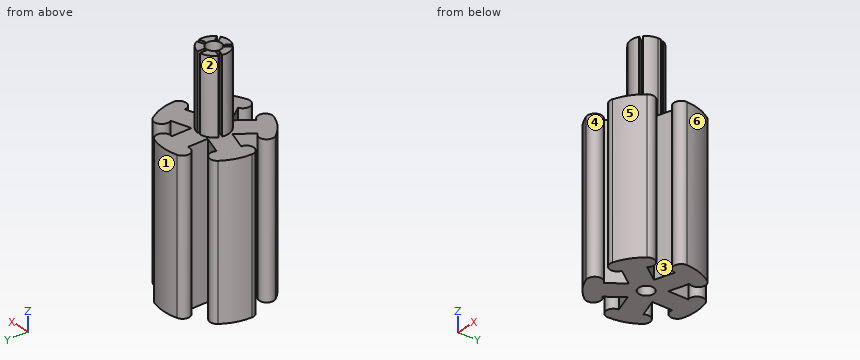
```python
from build123d import *

# Parameters (mm, degrees)
BOSS_EXTRUDE3_DEPTH = 30
CIRPATTERN1_COUNT   = 5
BOSS_EXTRUDE4_DEPTH = 15
SKETCH6_R           = 1.5
CUT_EXTRUDE1_DEPTH  = 80


with BuildPart() as part:
    # Sketch2 → Boss-Extrude3 (new body)
    with BuildSketch(Plane.XY):
        with BuildLine():
            Line((-2.054029869, 6.78303703), (-2.054029869, 0))
            Line((-2.054029869, 0), (2.054029869, 0))
            Line((2.054029869, 0), (2.054029869, 6.78303703))
            ThreePointArc((2.054029869, 6.78303703), (3.825708627, 7.801903653), (2.835284544, 9.589638239))
            ThreePointArc((2.835284544, 9.589638239), (0, 10), (-2.835284544, 9.589638239))
            ThreePointArc((-2.835284544, 9.589638239), (-3.825708627, 7.801903653), (-2.054029869, 6.78303703))
        make_face()
    extrude(amount=-BOSS_EXTRUDE3_DEPTH)

    # CirPattern1: part ×5 about axis
    cirpattern1_axis = Axis((0, 0, 0), (0, 0, 1))


with BuildPart() as part_1:
    add(part.part)
    for i in range(1, CIRPATTERN1_COUNT):
        add(part.part.rotate(cirpattern1_axis, i * 360 / CIRPATTERN1_COUNT))

    # Sketch7 → Boss-Extrude4 (add)
    with BuildSketch(Plane.XY):
        with BuildLine():
            Line((0.3, 2.984962311), (0.3, 1.687380928))
            Line((0.3, 1.687380928), (-0.3, 1.687380928))
            Line((-0.3, 1.687380928), (-0.3, 2.984962311))
            ThreePointArc((-0.3, 2.984962311), (-1.763355757, 2.427050983), (-2.746162759, 1.207721037))
            Line((-2.746162759, 1.207721037), (-1.512089528, 0.806746337))
            Line((-1.512089528, 0.806746337), (-1.697499725, 0.236112428))
            Line((-1.697499725, 0.236112428), (-2.931572955, 0.637087127))
            ThreePointArc((-2.931572955, 0.637087127), (-2.853169549, -0.927050983), (-1.997221924, -2.238549662))
            Line((-1.997221924, -2.238549662), (-1.234522723, -1.188784271))
            Line((-1.234522723, -1.188784271), (-0.749112526, -1.541455422))
            Line((-0.749112526, -1.541455422), (-1.511811727, -2.591220813))
            ThreePointArc((-1.511811727, -2.591220813), (0, -3), (1.511811727, -2.591220813))
            Line((1.511811727, -2.591220813), (0.749112526, -1.541455422))
            Line((0.749112526, -1.541455422), (1.234522723, -1.188784271))
            Line((1.234522723, -1.188784271), (1.997221924, -2.238549662))
            ThreePointArc((1.997221924, -2.238549662), (2.737851874, -1.226444909), (3, 0))
            ThreePointArc((3, 0), (2.982844185, 0.320375665), (2.931572955, 0.637087127))
            Line((2.931572955, 0.637087127), (1.697499725, 0.236112428))
            Line((1.697499725, 0.236112428), (1.512089528, 0.806746337))
            Line((1.512089528, 0.806746337), (2.746162759, 1.207721037))
            ThreePointArc((2.746162759, 1.207721037), (1.763355757, 2.427050983), (0.3, 2.984962311))
        make_face()
    extrude(amount=BOSS_EXTRUDE4_DEPTH)

    # Sketch6 → Cut-Extrude1 (cut)
    with BuildSketch(Plane(origin=(0, 0, -30), x_dir=(-1, 0, 0), z_dir=(0, 0, -1))):
        Circle(SKETCH6_R)
    extrude(amount=-CUT_EXTRUDE1_DEPTH, mode=Mode.SUBTRACT)


solid = part_1.part
```
Input: part model. Units: mm. Frame: model coordinates. Face numbers are marked on the shaded views. A direction names the side the tool comes from. Coordinates: 2 decimals unless noted, no trailing zeros. Order: outer loops, then holes, each group sorted by start corner. A loop starts at its lowest first (then second) coordinate and runs counter-clockwise, first axis right, second up. Notation, with made-up numbers: (52.5, 88) - (72.5, 88) arc R11 cw to (72.5, 101) - close; hole circle Ø6 at (-29.5, -12.75). An arc over 180 degrees is marked (long way). Put each result on its own line as item: value.
1. Line query: line 1 along Z through (x, y) = (5, 0.5); line 2 along X through (y, z) = (-4, -23.5); line 3 along Y through (x, z) = (3.25, -10). Output: solid intervals per line, ascending.
Report:
line 1: z = -30 to 0
line 2: x = -7.6 to -5.96, -5.45 to -0.37, 0.37 to 5.45, 5.96 to 7.6
line 3: y = -9.45 to 3.22, 6.99 to 9.39
2. Cut plane C-C on y = 7.25. Return the cut outline in (x, z), then the cut area to 3 significant figures.
Report:
outline: (-3.53, -30) - (3.53, -30) - (3.53, 0) - (-3.53, 0) - close
area: 212 mm2
3. Reachability of the marked faces 1, 2 and 3 from +Z, -Z, +X, -X, +Y, -Y: full face, straight path, thin tool, end or side. Return the list, or none.
Report:
face 1: +Z, -Z, +Y
face 2: +Z, -X, +Y
face 3: +Z, -Z
4. Cut plane D-D on x = 8.75. Return the cut outline in (y, z), then the cut area to 3 significant figures.
Report:
outline: (-1.21, -30) - (4.84, -30) - (4.84, 0) - (-1.21, 0) - close
area: 182 mm2
5. Contact query for flat-ended pins moving along their axis: pin 1 Ø10 at (x, z) = (6.5, -13.5) entering from +Y; pin 2 Ø3 at (y, z) = (5.5, -8) entering from -X; pin 3 Ø1 at (y, z) = (2.5, 9) entering from -X. Output: stop coordinate, or through.
Report:
pin 1: stops at y = 9.89
pin 2: stops at x = -9.17
pin 3: stops at x = -2.24
6. Cut plane A-A on z = 5. Return the cut outline in (x, y), then the cut area to 3 significant figures.
Report:
outline: (-2.93, 0.64) arc R3 ccw to (-2, -2.24) - (-1.23, -1.19) - (-0.75, -1.54) - (-1.51, -2.59) arc R3 ccw to (1.51, -2.59) - (0.75, -1.54) - (1.23, -1.19) - (2, -2.24) arc R3 ccw to (2.93, 0.64) - (1.7, 0.24) - (1.51, 0.81) - (2.75, 1.21) arc R3 ccw to (0.3, 2.98) - (0.3, 1.69) - (-0.3, 1.69) - (-0.3, 2.98) arc R3 ccw to (-2.75, 1.21) - (-1.51, 0.81) - (-1.7, 0.24) - close; hole circle Ø3 at (0, 0)
area: 17.3 mm2
7. Draft query along Y for the marked faces 4, 5 and 6. Return one class per face: pulls with the +Y half, pulls with the -Y half, needs draft (parallel to the pull), parting line crosses it, or undercut.
Report:
face 4: undercut
face 5: pulls with the -Y half
face 6: pulls with the +Y half
